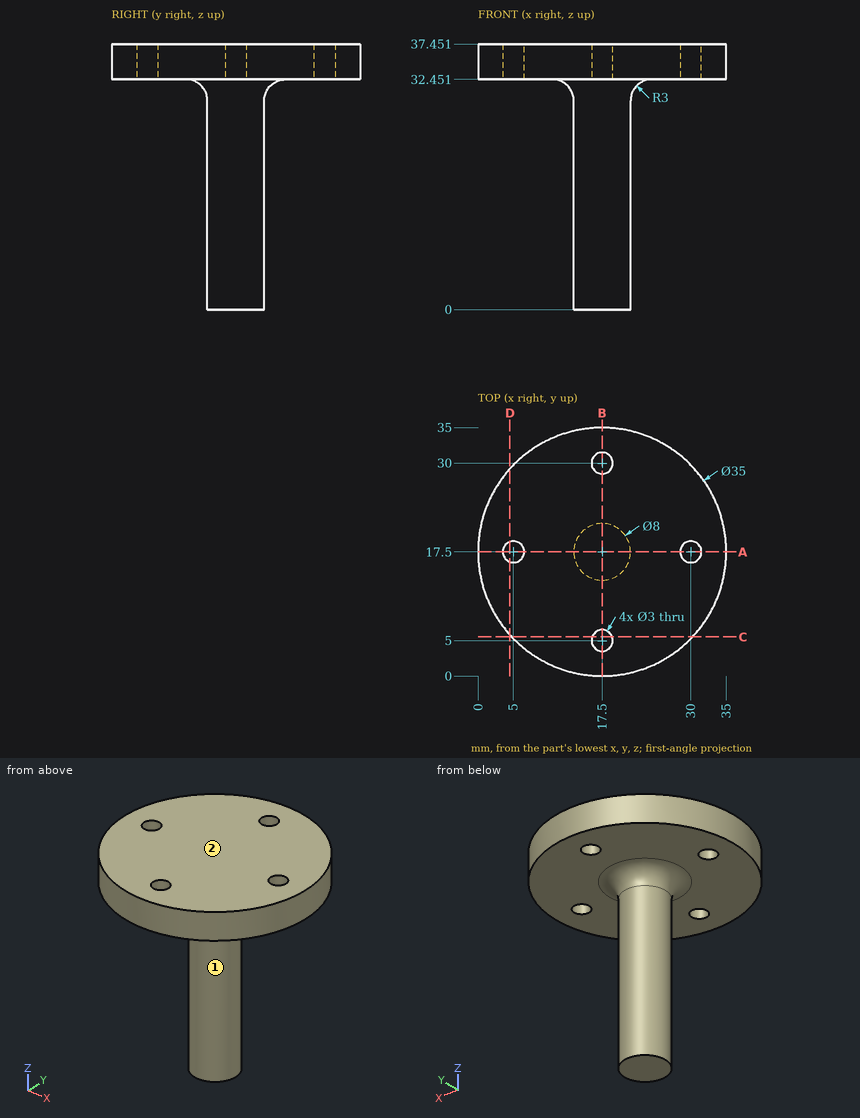
Answer from the drawing. Dimensions are ordinates in mm from the lowest x, y and z of the part. A direction names the side the tool comes from. Round coordinates to 2 decimals unless told otherwise and drop trailing zeros. Loops run counter-clockwise (first coordinate to the right, second up) from the corner with the lowest first, then second, coordinate; pieces in that order, holes last.
1) For the marked faces 1 and 2, determine the directions among +Z, -Z, +X, -X, +Y, -Y from which every point of the face is accessible in a straight line to the end or side of a thin tool.
Outcome:
face 1: -Z
face 2: +Z, +X, -X, +Y, -Y
2) Given P1, Ø1.5, axis at y = 23.5, z = 24.5, coming from the -X side; P2, Ø3.5, axis at x = 17.5, y = 5, coming from the -Z side; P3, Ø1.5, axis at x = 22.5, y = 21.5, coming from the -Z side; P4, Ø5, axis at x = 16.5, z = 15, coming from the -Y side, each flat-ended and moving along its own axis, determine where each tip first touches the part or whether it passes through.
Outcome:
P1: passes through
P2: stops at z = 32.45
P3: stops at z = 32.13
P4: stops at y = 13.5
3) A cutting plane is placed at C-C on y = 5.5. Determine the outline of the cut face in (x, z), plus the area to 3 significant figures.
Outcome:
outline: (4.76, 32.45) - (16.09, 32.45) - (16.09, 37.45) - (4.76, 37.45) - close; (18.91, 32.45) - (30.24, 32.45) - (30.24, 37.45) - (18.91, 37.45) - close
area: 113 mm2
4) Consider line 1 (Y direction, x = 17.5, z = 33.8); line 2 (X direction, y = 17, z = 35); line 3 (X direction, y = 18.5, z = 34). Determine where each line is inside the solid, lowest interval first.
Outcome:
line 1: y = 0 to 3.5, 6.5 to 28.5, 31.5 to 35
line 2: x = 0.01 to 3.59, 6.41 to 28.59, 31.41 to 34.99
line 3: x = 0.03 to 3.88, 6.12 to 28.88, 31.12 to 34.97
5) A cutting plane is placed at A-A on y = 17.5. Determine the outline of the cut face in (x, z), plus the area to 3 significant figures.
Outcome:
outline: (0, 32.45) - (3.5, 32.45) - (3.5, 37.45) - (0, 37.45) - close; (6.5, 32.45) - (10.5, 32.45) arc R3 cw to (13.5, 29.45) - (13.5, 0) - (21.5, 0) - (21.5, 29.45) arc R3 cw to (24.5, 32.45) - (28.5, 32.45) - (28.5, 37.45) - (6.5, 37.45) - close; (31.5, 32.45) - (35, 32.45) - (35, 37.45) - (31.5, 37.45) - close
area: 408 mm2
6) A cutting plane is placed at D-D on x = 4.5. Determine the outline of the cut face in (y, z).
Outcome:
outline: (5.78, 32.45) - (16.09, 32.45) - (16.09, 37.45) - (5.78, 37.45) - close; (18.91, 32.45) - (29.22, 32.45) - (29.22, 37.45) - (18.91, 37.45) - close
